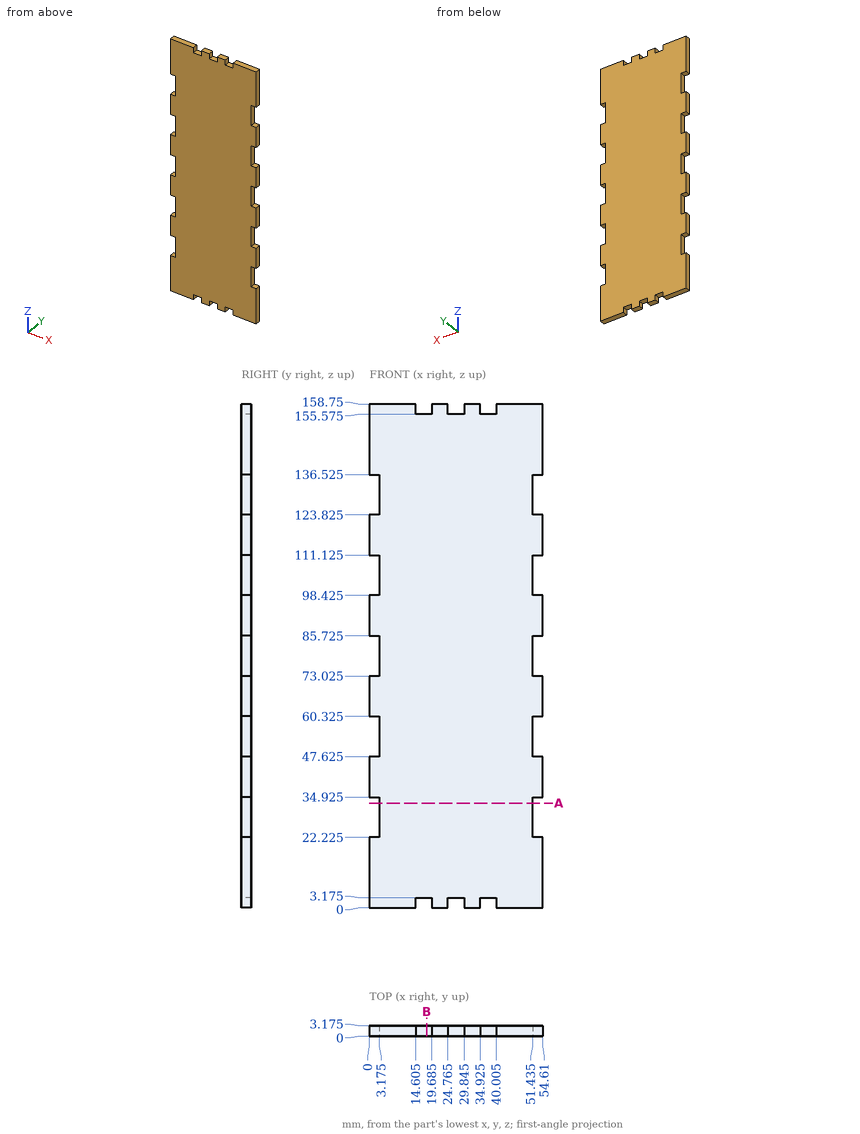
Print and shaded views of the part. All mm, measured from the part's lowest x, y and z. Round coordinates to 2 decimals unless told otherwise and drop trailing zeros. Write each loop counter-clockwise with the first axis right and the second up, starting at its lowest first coordinate (ties: lowest second). Pieces come first, ordered by that corner, then holes. Notation, with made-up numbers: (64, 45) - (95, 45) arc R29 cw to (95, 78) - close; hole circle Ø11 at (-18, 19). An arc over 180 degrees is marked (long way). One line per question, with ' | ' between items.
1. Band-saw the part on A-A, the plane z = 33. Write the cut outline in (x, y) (3 decimals), and give its area (3 significant figures).
Results are:
outline: (3.175, 0) - (51.435, 0) - (51.435, 3.175) - (3.175, 3.175) - close | area: 153 mm^2
2. Band-saw the part on B-B, the plane x = 18. Write the cut outline in (y, z) (3 decimals), and give its area (3 significant figures).
Results are:
outline: (0, 3.175) - (3.175, 3.175) - (3.175, 155.575) - (0, 155.575) - close | area: 484 mm^2
3. Drop flat-ended pins along their axis: pin 1 Ø1.5 at (x, y) = (16, 0.5) entering from +Z (3 decimals); pin 2 Ø1 at (y, z) = (1.5, 53.5) entering from -X (3 decimals). Give the stop position or say it passes through.
Results are:
pin 1: z = 155.575 | pin 2: x = 3.175
4. Drill centre lines: line 1 along X through (y, z) = (1.7, 28.5) (3 decimals); line 2 along Z through (x, y) = (37.5, 2.6) (3 decimals). Where is each one in solid material? Low to high. Write a range as from..to.
Results are:
line 1: 3.175..51.435 | line 2: 3.175..155.575
